Design review of the part built by this model. Coordinates are the model's own, in mm. Give positions to 0.01 mm unless a question says otherwise; leave off trailing zeros. Loops run counter-clockwise (first coordinate to the right, second up) from the corner with the lowest first, then second, coordinate; pieces in that order, holes last. Notation, with made-up numbers: (-11, 26.25) -> (29, 26.25) arc R23 cw to (29, 58.25) -> close; hole circle Ø1 at (-36.75, -8.5). An arc over 180 degrees is marked (long way). Use a Markdown table: item, result. Add a question column.
1. To check wall thickness, follow line 1 (X direction, y = -7.2, z = 5); line 2 (X direction, y = -10.8, z = 2.5); line 3 (X direction, y = -26, z = 2). State the ranges of each line that lie inside material, in increasing order.
2. Draft analysis for pull direction Y (two halves, no side actions). For faces 1 (the cylindrical face through (15.622, -3.495, 5.07)), 2 (the flat face through (0, 0, 10)), state which applies: pulls with the +Y half, pulls with the -Y half, needs draft (parallel to the pull), parting line crosses it, or undercut.
3. Add section B-B (y = 10.8). State the section outline as (x, z) points, and give its area (3 significant figures).
4. Add section A-A (x = 0). State the section outline as (y, z) points, and give its area (3 significant figures).
5. Add section D-D (x = 12.5). Count the separate pieces of the cut face and the enclosed holes in it, and give its area (3 significant figures).
6. Add section C-C (y = 21.6). State the section outline as (x, z) points.
7. For pin 1 Ø4 at (x, y) = (-12, 14.4) entering from +Z, flat-tipped, find the tip position at first contact; note if it passes through.
Autodesk Inventor part; units mm, degrees
ref_plane "Work Plane2" through (-30, 0, 0) normal (0, 1, 0) x (1, 0, 0)
ref_plane "Work Plane1" through (-30, 0, 0) normal (0, 1, 0) x (1, 0, 0)
ref_plane "YZ Plane" through (0, 0, 0) normal (1, 0, 0) x (0, 1, 0)
sketch "Sketch1" plane through (0, 0, 0) normal (0, 0, 1) x (1, 0, 0)
  line L0 (-30, -30) -> (30, -30)
  line L1 (30, -30) -> (30, 30)
  line L2 (30, 30) -> (-30, 30)
  line L3 (-30, 30) -> (-30, -30)
  line L4 (-30, -30) -> (30, 30) construction
  line L5 (30, -30) -> (-30, 30) construction
  point P0 (0, 0)
  dimension "d0" = 60
  dimension "d1" = 60
extrude "Extrusion1" add sketch "Sketch1" along normal blind 10
sketch "Sketch3" plane through (0, 0, 10) normal (0, 0, 1) x (1, 0, 0)
  circle A0 centre (0, 0) radius 29
  line L0 (-14.3513, 25.2) -> (14.3513, 25.2) construction
  line L1 (-19.3505, 21.6) -> (19.3505, 21.6) construction
  line L2 (22.7376, 18) -> (-22.7376, 18) construction
  line L3 (-25.1722, 14.4) -> (25.1722, 14.4) construction
  line L4 (26.9139, 10.8) -> (-26.9139, 10.8) construction
  line L5 (-28.092, 7.2) -> (28.092, 7.2) construction
  line L6 (28.7757, 3.6) -> (-28.7757, 3.6) construction
  line L7 (-29, 0) -> (29, 0) construction
  circle A1 centre (-5, 25.2) radius 2.38
  circle A2 centre (5, 25.2) radius 2.38
  circle A3 centre (-12, 21.6) radius 2.38
  circle A4 centre (0, 21.6) radius 2.38
  circle A5 centre (12, 21.6) radius 2.38
  circle A6 centre (-17.5, 18) radius 2.38
  circle A7 centre (-6, 18) radius 2.38
  circle A8 centre (6, 18) radius 2.38
  circle A9 centre (17.5, 18) radius 2.38
  circle A10 centre (-12, 14.4) radius 2.38
  circle A11 centre (0, 14.4) radius 2.38
  circle A12 centre (12, 14.4) radius 2.38
  circle A13 centre (-19, 10.8) radius 2.38
  circle A14 centre (19, 10.8) radius 2.38
  circle A15 centre (6, 10.8) radius 2.38
  circle A16 centre (-6, 10.8) radius 2.38
  circle A17 centre (-24, 7.2) radius 2.38
  circle A18 centre (-12.5, 7.2) radius 2.38
  circle A19 centre (0, 7.2) radius 2.38
  circle A20 centre (12.5, 7.2) radius 2.38
  circle A21 centre (24, 7.2) radius 2.38
  circle A22 centre (-18, 3.6) radius 2.38
  circle A23 centre (-6, 3.6) radius 2.38
  circle A24 centre (6, 3.6) radius 2.38
  circle A25 centre (18, 3.6) radius 2.38
  circle A26 centre (-24.5, 0) radius 2.38
  circle A27 centre (-12, 0) radius 2.38
  circle A28 centre (12, 0) radius 2.38
  circle A29 centre (24.5, 0) radius 2.38
  dimension "d52" = 58
  dimension "d53" = 3.6
  dimension "d54" = 3.6
  dimension "d55" = 3.6
  dimension "d56" = 3.6
  dimension "d57" = 3.6
  dimension "d58" = 3.6
  dimension "d59" = 3.6
  dimension "d65" = 5
  dimension "d66" = 5
  dimension "d67" = 4.76
  dimension "d68" = 12
  dimension "d69" = 12
  dimension "d70" = 6
  dimension "d71" = 6
  dimension "d72" = 17.5
  dimension "d73" = 17.5
  dimension "d74" = 12
  dimension "d75" = 12
  dimension "d76" = 19
  dimension "d77" = 6
  dimension "d78" = 6
  dimension "d79" = 19
  dimension "d80" = 12.5
  dimension "d81" = 12.5
  dimension "d82" = 24
  dimension "d83" = 24
  dimension "d84" = 6
  dimension "d85" = 6
  dimension "d86" = 18
  dimension "d87" = 18
  dimension "d88" = 12
  dimension "d89" = 12
  dimension "d90" = 24.5
  dimension "d91" = 24.5
extrude "Extrusion3" cut sketch "Sketch3" against normal up to next contours A1 | A2 | A3 | A4 | A5 | A6 | A7 | A8 | A9 | A10 | A11 | A12 | A13 | A14 | A15 | A16 | A17 | A18 | A19 | A20 | A21 | A22 | A23 | A24 | A25 | A26 | A27 | A28 | A29
ref_plane "Work Plane2" through (-30, 0, 0) normal (0, 1, 0) x (1, 0, 0)
mirror "Mirror2" about plane through (-30, 0, 0) normal (0, 1, 0) of "Extrusion3"
sketch "Sketch2" plane through (0, 0, 10) normal (0, 0, 1) x (1, 0, 0)
  circle A0 centre (0, 0) radius 29
  line L0 (-18.8944, 22) -> (18.8944, 22) construction
  line L1 (-21.9089, 19) -> (21.9089, 19) construction
  line L2 (-24.1868, 16) -> (24.1868, 16) construction
  line L3 (-25.923, 13) -> (-25.923, 13) construction
  line L4 (-25.923, 13) -> (25.923, 13) construction
  line L5 (-27.2213, 10) -> (27.2213, 10) construction
  line L6 (-7.5498, 28) -> (7.5498, 28) construction
  line L7 (-14.6969, 25) -> (14.6969, 25) construction
  line L8 (-28.2622, 6.5) -> (28.2622, 6.5) construction
  line L9 (-28.8444, 3) -> (28.8444, 3) construction
  line L10 (-29, 0) -> (29, 0) construction
  circle A1 centre (0, 25) radius 2.38
  circle A2 centre (-10, 25) radius 2.38
  circle A3 centre (10, 25) radius 2.38
  circle A4 centre (5, 22) radius 2.38
  circle A5 centre (14.5, 22) radius 2.38
  circle A6 centre (-5, 22) radius 2.38
  circle A7 centre (-14.5, 22) radius 2.38
  circle A8 centre (-10, 19) radius 2.38
  circle A9 centre (-19, 19) radius 2.38
  circle A10 centre (0, 19) radius 2.38
  circle A11 centre (10, 19) radius 2.38
  circle A12 centre (19, 19) radius 2.38
  circle A13 centre (-14.5, 16) radius 2.38
  circle A14 centre (-5, 16) radius 2.38
  circle A15 centre (5, 16) radius 2.38
  circle A16 centre (14.5, 16) radius 2.38
  circle A17 centre (-19.5, 13) radius 2.38
  circle A18 centre (-10, 13) radius 2.38
  circle A19 centre (0, 13) radius 2.38
  circle A20 centre (10, 13) radius 2.38
  circle A21 centre (19.5, 13) radius 2.38
  circle A22 centre (-24, 10) radius 2.38
  circle A23 centre (-15, 10) radius 2.38
  circle A24 centre (-5, 10) radius 2.38
  circle A25 centre (5, 10) radius 2.38
  circle A26 centre (15, 10) radius 2.38
  circle A27 centre (24, 10) radius 2.38
  circle A28 centre (-19.5, 6.5) radius 2.38
  circle A29 centre (-10, 6.5) radius 2.38
  circle A30 centre (0, 6.5) radius 2.38
  circle A31 centre (10, 6.5) radius 2.38
  circle A32 centre (19.5, 6.5) radius 2.38
  circle A33 centre (-25, 3) radius 2.38
  circle A34 centre (-15, 3) radius 2.38
  circle A35 centre (-5, 3) radius 2.38
  circle A36 centre (5, 3) radius 2.38
  circle A37 centre (15, 3) radius 2.38
  circle A38 centre (25, 3) radius 2.38
  circle A39 centre (-20, 0) radius 2.38
  circle A40 centre (-10, 0) radius 2.38
  circle A41 centre (10, 0) radius 2.38
  circle A42 centre (20, 0) radius 2.38
  dimension "d4" = 58
  dimension "d5" = 3
  dimension "d6" = 3
  dimension "d7" = 3
  dimension "d8" = 3
  dimension "d9" = 3.5
  dimension "d10" = 3.5
  dimension "d11" = 3
  dimension "d12" = 3
  dimension "d13" = 3
  dimension "d14" = 4.76
  dimension "d15" = 10
  dimension "d16" = 10
  dimension "d17" = 14.5
  dimension "d18" = 5
  dimension "d19" = 5
  dimension "d20" = 14.5
  dimension "d21" = 10
  dimension "d22" = 19
  dimension "d23" = 19
  dimension "d24" = 10
  dimension "d25" = 5
  dimension "d26" = 5
  dimension "d27" = 14.5
  dimension "d28" = 14.5
  dimension "d29" = 10
  dimension "d30" = 10
  dimension "d31" = 19.5
  dimension "d32" = 19.5
  dimension "d33" = 24
  dimension "d34" = 24
  dimension "d35" = 15
  dimension "d36" = 15
  dimension "d37" = 5
  dimension "d38" = 5
  dimension "d39" = 5
  dimension "d40" = 5
  dimension "d41" = 15
  dimension "d42" = 25
  dimension "d43" = 25
  dimension "d44" = 15
  dimension "d45" = 20
  dimension "d46" = 10
  dimension "d47" = 10
  dimension "d48" = 20
properties part number "FanTemplate60mm"
Taken from the geometry:
| question | item | result |
|---|---|---|
| 1 | line 1 | x = -30 to -26.38, -21.62 to -14.88, -10.12 to -2.38, 2.38 to 10.12, 14.88 to 21.62, 26.38 to 30 |
| 1 | line 2 | x = -30 to -21.38, -16.62 to -8.38, -3.62 to 3.62, 8.38 to 16.62, 21.38 to 30 |
| 1 | line 3 | x = -30 to -7.24, -2.76 to 2.76, 7.24 to 30 |
| 2 | face 1 | undercut |
| 2 | face 2 | needs draft |
| 3 | outline | (-30, 0) -> (-21.38, 0) -> (-21.38, 10) -> (-30, 10) -> close; (-16.62, 0) -> (-8.38, 0) -> (-8.38, 10) -> (-16.62, 10) -> close; (-3.62, 0) -> (3.62, 0) -> (3.62, 10) -> (-3.62, 10) -> close; (8.38, 0) -> (16.62, 0) -> (16.62, 10) -> (8.38, 10) -> close; (21.38, 0) -> (30, 0) -> (30, 10) -> (21.38, 10) -> close |
| 3 | area | 410 mm^2 |
| 4 | outline | (-30, 0) -> (-23.98, 0) -> (-23.98, 10) -> (-30, 10) -> close; (-19.22, 0) -> (-16.78, 0) -> (-16.78, 10) -> (-19.22, 10) -> close; (-12.02, 0) -> (-9.58, 0) -> (-9.58, 10) -> (-12.02, 10) -> close; (-4.82, 0) -> (4.82, 0) -> (4.82, 10) -> (-4.82, 10) -> close; (9.58, 0) -> (12.02, 0) -> (12.02, 10) -> (9.58, 10) -> close; (16.78, 0) -> (19.22, 0) -> (19.22, 10) -> (16.78, 10) -> close; (23.98, 0) -> (30, 0) -> (30, 10) -> (23.98, 10) -> close |
| 4 | area | 314 mm^2 |
| 5 | separate pieces | 8 |
| 5 | enclosed holes | 0 |
| 5 | area | 272 mm^2 |
| 6 | outline | (-30, 0) -> (-14.38, 0) -> (-14.38, 10) -> (-30, 10) -> close; (-9.62, 0) -> (-2.38, 0) -> (-2.38, 10) -> (-9.62, 10) -> close; (2.38, 0) -> (9.62, 0) -> (9.62, 10) -> (2.38, 10) -> close; (14.38, 0) -> (30, 0) -> (30, 10) -> (14.38, 10) -> close |
| 7 | pin 1 | passes through |
